Check sheet for the modelled part. Datum: model origin and axes. Units: mm. A direction names the side the tool comes from. Round coordinates to 2 decimals unless told otherwise and drop trailing zeros. Write each loop counter-clockwise with the first axis right and the second up, starting at its lowest first coordinate (ties: lowest second). Pieces come first, ordered by that corner, then holes. Notation, with made-up numbers: M 47,8 L 79,8 A24 ccw 79,44 Z; hole C 26.5,4.25 d11. An arc over 180 degrees is marked long. One line per item, written item: value.
from build123d import *

# Parameters (mm, degrees)
SKETCH1_W                                           = 110
SKETCH1_H                                           = 225
BOSS_EXTRUDE1_DEPTH                                 = 20
CUT_EXTRUDE1_REACH                                  = 128.812
CUT_EXTRUDE2_REACH                                  = 128.812
SKETCH4_R                                           = 10
CUT_EXTRUDE3_DEPTH                                  = 127.81186853
CUT_EXTRUDE4_REACH                                  = 128.812
SKETCH5_R                                           = 6
CUT_EXTRUDE5_REACH                                  = 128.812
SKETCH6_R                                           = 7
CBORE_FOR_M8_HEX_SOCKET_HEAD_CAP_SCREW1_D           = 8.4
CBORE_FOR_M8_HEX_SOCKET_HEAD_CAP_SCREW1_CBORE_D     = 15
CBORE_FOR_M8_HEX_SOCKET_HEAD_CAP_SCREW1_CBORE_DEPTH = 8.6
F_8_0MM_DOWEL_HOLE1_D                               = 8


with BuildPart() as part:
    # Sketch1 → Boss-Extrude1 (new body)
    with BuildSketch(Plane(origin=(0, 0, 0), x_dir=(1, 0, 0), z_dir=(0, 1, 0))):
        Rectangle(SKETCH1_W, SKETCH1_H)
    extrude(amount=BOSS_EXTRUDE1_DEPTH)

    # Sketch2 → Cut-Extrude1 (cut, up to next)
    with BuildSketch(Plane(origin=(0, 20, 0), x_dir=(1, 0, 0), z_dir=(0, 1, 0)), mode=Mode.PRIVATE) as cut_extrude1_sk1:
        with BuildLine():
            Line((-42.5, -32.64), (-22, -32.64))
            ThreePointArc((-22, -32.64), (-19.878679656, -31.761320344), (-19, -29.64))
            Line((-19, -29.64), (-19, -14.14))
            ThreePointArc((-19, -14.14), (-19.439339828, -13.079339828), (-20.5, -12.64))
            Line((-20.5, -12.64), (-34.5, -12.64))
            ThreePointArc((-34.5, -12.64), (-38.742640687, -10.882640687), (-40.5, -6.64))
            Line((-40.5, -6.64), (-40.5, 26.36))
            ThreePointArc((-40.5, 26.36), (-38.742640687, 30.602640687), (-34.5, 32.36))
            Line((-34.5, 32.36), (-20.5, 32.36))
            ThreePointArc((-20.5, 32.36), (-19.439339828, 32.799339828), (-19, 33.86))
            Line((-19, 33.86), (-19, 49.36))
            ThreePointArc((-19, 49.36), (-19.878679656, 51.481320344), (-22, 52.36))
            Line((-22, 52.36), (-42.5, 52.36))
            ThreePointArc((-42.5, 52.36), (-44.621320344, 51.481320344), (-45.5, 49.36))
            Line((-45.5, 49.36), (-45.5, -29.64))
            ThreePointArc((-45.5, -29.64), (-44.621320344, -31.761320344), (-42.5, -32.64))
        make_face()
    cut_extrude1_tool1 = extrude(cut_extrude1_sk1.sketch, amount=-CUT_EXTRUDE1_REACH, mode=Mode.PRIVATE) & part.part
    add(cut_extrude1_tool1.solids().sort_by_distance((-43.991747, 20, -50.851747))[0], mode=Mode.SUBTRACT)

    # Sketch3 → Cut-Extrude2 (cut, up to next)
    with BuildSketch(Plane(origin=(0, 20, 0), x_dir=(1, 0, 0), z_dir=(0, 1, 0)), mode=Mode.PRIVATE) as cut_extrude2_sk1:
        with BuildLine():
            Line((22, -8.64), (27.5, -8.64))
            ThreePointArc((27.5, -8.64), (28.914213562, -8.054213562), (29.5, -6.64))
            Line((29.5, -6.64), (29.5, 11.36))
            ThreePointArc((29.5, 11.36), (28.914213562, 12.774213562), (27.5, 13.36))
            Line((27.5, 13.36), (22, 13.36))
            ThreePointArc((22, 13.36), (19.878679656, 14.238679656), (19, 16.36))
            Line((19, 16.36), (19, 30.36))
            ThreePointArc((19, 30.36), (19.878679656, 32.481320344), (22, 33.36))
            Line((22, 33.36), (31.5, 33.36))
            ThreePointArc((31.5, 33.36), (33.621320344, 32.481320344), (34.5, 30.36))
            Line((34.5, 30.36), (34.5, -25.64))
            ThreePointArc((34.5, -25.64), (33.621320344, -27.761320344), (31.5, -28.64))
            Line((31.5, -28.64), (22, -28.64))
            ThreePointArc((22, -28.64), (19.878679656, -27.761320344), (19, -25.64))
            Line((19, -25.64), (19, -11.64))
            ThreePointArc((19, -11.64), (19.878679656, -9.518679656), (22, -8.64))
        make_face()
    cut_extrude2_tool1 = extrude(cut_extrude2_sk1.sketch, amount=-CUT_EXTRUDE2_REACH, mode=Mode.PRIVATE) & part.part
    add(cut_extrude2_tool1.solids().sort_by_distance((24.75, 20, 9.279081))[0], mode=Mode.SUBTRACT)

    # Sketch4 → Cut-Extrude3 (cut, through all)
    with BuildSketch(Plane.XZ):
        with Locations(Location((37.5, 52.64, 0), (0, 0, 270))):
            Circle(SKETCH4_R)
        with Locations(Location((12.5, 52.64, 0), (0, 0, 270))):
            Circle(SKETCH4_R)
        with Locations(Location((-12.5, 52.64, 0), (0, 0, 270))):
            Circle(SKETCH4_R)
        with Locations(Location((-37.5, 52.64, 0), (0, 0, 270))):
            Circle(SKETCH4_R)
        with Locations(Location((0, 10.14, 0), (0, 0, 270))):
            Circle(SKETCH4_R)
        with Locations(Location((0, -29.86, 0), (0, 0, 270))):
            Circle(SKETCH4_R)
        with Locations(Location((37.5, -72.36, 0), (0, 0, 270))):
            Circle(SKETCH4_R)
        with Locations(Location((12.5, -72.36, 0), (0, 0, 270))):
            Circle(SKETCH4_R)
        with Locations(Location((-12.5, -72.36, 0), (0, 0, 270))):
            Circle(SKETCH4_R)
        with Locations(Location((-37.5, -72.36, 0), (0, 0, 270))):
            Circle(SKETCH4_R)
    extrude(amount=-CUT_EXTRUDE3_DEPTH, mode=Mode.SUBTRACT)

    # Sketch5 → Cut-Extrude4 (cut, up to next)
    with BuildSketch(Plane(origin=(0, 20, 0), x_dir=(1, 0, 0), z_dir=(0, 1, 0)), mode=Mode.PRIVATE) as cut_extrude4_sk1:
        with Locations(Location((-37.5, 92.36, 0), (0, 0, 270))):
            Circle(SKETCH5_R)
    cut_extrude4_tool1 = extrude(cut_extrude4_sk1.sketch, amount=-CUT_EXTRUDE4_REACH, mode=Mode.PRIVATE) & part.part
    # Sketch5 → Cut-Extrude4 (cut, up to next)
    with BuildSketch(Plane(origin=(0, 20, 0), x_dir=(1, 0, 0), z_dir=(0, 1, 0)), mode=Mode.PRIVATE) as cut_extrude4_sk2:
        with Locations(Location((37.5, 92.36, 0), (0, 0, 270))):
            Circle(SKETCH5_R)
    cut_extrude4_tool2 = extrude(cut_extrude4_sk2.sketch, amount=-CUT_EXTRUDE4_REACH, mode=Mode.PRIVATE) & part.part
    # Sketch5 → Cut-Extrude4 (cut, up to next)
    with BuildSketch(Plane(origin=(0, 20, 0), x_dir=(1, 0, 0), z_dir=(0, 1, 0)), mode=Mode.PRIVATE) as cut_extrude4_sk3:
        with Locations(Location((-37.5, -72.64, 0), (0, 0, 270))):
            Circle(SKETCH5_R)
    cut_extrude4_tool3 = extrude(cut_extrude4_sk3.sketch, amount=-CUT_EXTRUDE4_REACH, mode=Mode.PRIVATE) & part.part
    # Sketch5 → Cut-Extrude4 (cut, up to next)
    with BuildSketch(Plane(origin=(0, 20, 0), x_dir=(1, 0, 0), z_dir=(0, 1, 0)), mode=Mode.PRIVATE) as cut_extrude4_sk4:
        with Locations(Location((37.5, -72.64, 0), (0, 0, 270))):
            Circle(SKETCH5_R)
    cut_extrude4_tool4 = extrude(cut_extrude4_sk4.sketch, amount=-CUT_EXTRUDE4_REACH, mode=Mode.PRIVATE) & part.part
    add(cut_extrude4_tool1.solids().sort_by_distance((-37.5, 20, -92.36))[0], mode=Mode.SUBTRACT)
    add(cut_extrude4_tool2.solids().sort_by_distance((37.5, 20, -92.36))[0], mode=Mode.SUBTRACT)
    add(cut_extrude4_tool3.solids().sort_by_distance((-37.5, 20, 72.64))[0], mode=Mode.SUBTRACT)
    add(cut_extrude4_tool4.solids().sort_by_distance((37.5, 20, 72.64))[0], mode=Mode.SUBTRACT)

    # Sketch6 → Cut-Extrude5 (cut, up to next)
    with BuildSketch(Plane(origin=(0, 20, 0), x_dir=(1, 0, 0), z_dir=(0, 1, 0)), mode=Mode.PRIVATE) as cut_extrude5_sk1:
        with Locations(Location((0, 9.86, 0), (0, 0, 270))):
            Circle(SKETCH6_R)
    cut_extrude5_tool1 = extrude(cut_extrude5_sk1.sketch, amount=-CUT_EXTRUDE5_REACH, mode=Mode.PRIVATE) & part.part
    add(cut_extrude5_tool1.solids().sort_by_distance((0, 20, -9.86))[0], mode=Mode.SUBTRACT)

    # CBORE for M8 Hex Socket Head Cap Screw1 (through all)
    with Locations(Plane(origin=(0, 0, 0), x_dir=(-1, 0, 0), z_dir=(0, -1, 0))):
        with Locations((-17, 96.5), (17, 96.5), (-39, -96.5), (39, -96.5)):
            CounterBoreHole(CBORE_FOR_M8_HEX_SOCKET_HEAD_CAP_SCREW1_D / 2, CBORE_FOR_M8_HEX_SOCKET_HEAD_CAP_SCREW1_CBORE_D / 2, CBORE_FOR_M8_HEX_SOCKET_HEAD_CAP_SCREW1_CBORE_DEPTH)

    # Ø8.0mm Dowel Hole1 (through all)
    with Locations(Plane(origin=(0, 0, 0), x_dir=(-1, 0, 0), z_dir=(0, -1, 0))):
        with Locations((0, 96.5), (-23.5, -96.5), (23.5, -96.5)):
            Hole(F_8_0MM_DOWEL_HOLE1_D / 2)


solid = part.part
Q1. Sectioned sample at C-C on y = 10.75. State how many separate pieces and enclosed holes the cut face has, and give its area (3 significant figures).
Completed:
separate pieces: 1
enclosed holes: 24
area: 18,600 mm^2
Q2. Sectioned sample at B-B on x = 0. Enter the section's corners in (y, z), and give its area (3 significant figures).
Completed:
outline: M 0,-112.5 L 20,-112.5 L 20,-100.5 L 0,-100.5 Z; M 0,-92.5 L 20,-92.5 L 20,-39.86 L 0,-39.86 Z; M 0,-19.86 L 20,-19.86 L 20,-16.86 L 0,-16.86 Z; M 0,-2.86 L 20,-2.86 L 20,0.14 L 0,0.14 Z; M 0,20.14 L 20,20.14 L 20,112.5 L 0,112.5 Z
area: 3,260 mm^2
Q3. Depth check by flat-ended pin: P1, Ø11, axis at x = 39, z = 96.5, coming from the -Y side. Enter the tip coordinate at first touch or a pass-through.
Completed:
P1: y = 8.6
Q4. Sectioned sample at A-A on z = -72.36. Enter the section's corners in (x, y), and give its area (3 significant figures).
Completed:
outline: M -55,0 L -47.5,0 L -47.5,20 L -55,20 Z; M -27.5,0 L -22.5,0 L -22.5,20 L -27.5,20 Z; M -2.5,0 L 2.5,0 L 2.5,20 L -2.5,20 Z; M 22.5,0 L 27.5,0 L 27.5,20 L 22.5,20 Z; M 47.5,0 L 55,0 L 55,20 L 47.5,20 Z
area: 600 mm^2
Q5. Scan lines: line 1 (X direction, y = 12, z = -9.86); line 2 (Z direction, x = -23.5, y = 11); line 3 (X direction, y = 6.25, z = 96.5). Record each from-to range of solid material in increasing order. Write a range as [from, to].
Completed:
line 1: [-55, -45.5], [-40.5, -7], [7, 29.5], [34.5, 55]
line 2: [-112.5, -52.36], [-32.36, 12.64], [32.64, 92.5], [100.5, 112.5]
line 3: [-55, -46.5], [-31.5, -27.5], [-19.5, 19.5], [27.5, 31.5], [46.5, 55]
Q6. Access from +Z, -Z, +X, -X, +Y, -Y to the whole of each face (thin tool, end or side, straight path). Record for faces 1 (the cylindrical face through (-37.37, 4.24, 103.82)), 2 (the flat face through (25, 10, -13.36)).
Completed:
face 1: -Y
face 2: +Y, -Y
Q7. Sectioned sample at D-D on x = -16. Enter the section's corners in (y, z), and give its area (3 significant figures).
Completed:
outline: M 0,-112.5 L 20,-112.5 L 20,-100.58 L 8.6,-100.58 L 8.6,-103.93 L 0,-103.93 Z; M 0,-89.07 L 8.6,-89.07 L 8.6,-92.42 L 20,-92.42 L 20,-81.73 L 0,-81.73 Z; M 0,-62.99 L 20,-62.99 L 20,43.27 L 0,43.27 Z; M 0,62.01 L 20,62.01 L 20,112.5 L 0,112.5 Z
area: 3,530 mm^2
